Autodesk Inventor part; units mm, degrees
ref_plane "YZ Plane" through (0, 0, 0) normal (1, 0, 0) x (0, 1, 0)
ref_plane "XZ Plane" through (0, 0, 0) normal (0, 1, 0) x (-1, 0, 0)
ref_plane "XY Plane" through (0, 0, 0) normal (0, 0, 1) x (1, 0, 0)
sketch "草圖1" plane through (0, 0, 0) normal (0, 1, 0) x (-1, 0, 0)
  line L0 (-14.2, 4) -> (14.2, 4)
  line L1 (14.2, 4) -> (14.2, -4)
  line L2 (-14.2, -4) -> (-14.2, 4)
  line L3 (-14.2, 4) -> (14.2, -4) construction
  line L4 (14.2, 4) -> (-14.2, -4) construction
  line L5 (-11.2, -4) -> (-11.2, 0)
  line L6 (-11.2, 0) -> (-8.2, 0)
  line L7 (-8.2, 0) -> (-8.2, -4)
  line L8 (0, 7.3969) -> (0, -7.2649)
  line L9 (11.2, -4) -> (11.2, 0)
  line L10 (11.2, 0) -> (8.2, 0)
  line L11 (8.2, 0) -> (8.2, -4)
  line L12 (14.2, -4) -> (11.2, -4)
  line L13 (8.2, -4) -> (-8.2, -4)
  line L14 (-11.2, -4) -> (-14.2, -4)
  point P0 (0, 0)
  dimension "d0" = 4
  dimension "d1" = 8
  dimension "d2" = 16.4
  dimension "d3" = 3
  dimension "d5" = 28.4
extrude "擠出1" add sketch "草圖1" along normal blind 3
equation "\"d5\" = d2 + 4 * d3"
properties part number "upper support"
Could you check a few things on this model? Use its own coordinates, in mm. A direction names the side the tool comes from. Give positions to 0.01 mm unless a question says otherwise; leave off trailing zeros. Write each loop counter-clockwise with the first axis right and the second up, starting at its lowest first coordinate (ties: lowest second). Pieces come first, ordered by that corner, then holes. Notation, with made-up numbers: (17.5, 52.25) -> (39.5, 52.25) arc R20 cw to (39.5, 88.25) -> close; hole circle Ø4 at (72.25, 52). An arc over 180 degrees is marked (long way). Write each question's results on one line, items separated by ' | '. Start each with the question number.
Q1. Suppose I cut it at B-B, the plane y = 2.55. List the corners of the cut face in (x, z) for me, and give its area (3 significant figures).
Q2. Which directions (+Z, -Z, +X, -X, +Y, -Y) give clear straight access to the entire face, cutting with the end or side of a thin tool? Please do faces 4 (the face through (-13, 1, -4)), 5 (the face through (-11.2, 1, -2)).
Q3. We'd pull the mould along X, two halves only. Please class faces 1 (the face through (8.2, 1, -2)), 2 (the face through (0, 3, 0)), 3 (the face through (14.2, 1, 0)): +X half, -X half, draft (parallel to the pull), parting line (faces both ways), or undercut.
Q4. Suppose I cut it at C-C, the plane x = -10. List the corners of the cut face in (y, z) for me, and give its area (3 significant figures).
Q5. Suppose I cut it at A-A, the plane z = -2.25. List the corners of the cut face in (x, y) for me.
Q6. I need wall thicknesses on probe 1 along X at (y, z) = (0.85, -2.5); probe 2 along Z at (x, y) = (9, 2.4). Which ranges of each line are inside material? Lowest first, please.
Outcome:
1) outline: (-14.2, -4) -> (-11.2, -4) -> (-11.2, 0) -> (-8.2, 0) -> (-8.2, -4) -> (8.2, -4) -> (8.2, 0) -> (11.2, 0) -> (11.2, -4) -> (14.2, -4) -> (14.2, 4) -> (-14.2, 4) -> close | area: 203 mm2
2) face 4: -Z, +X, -X, +Y, -Y | face 5: -Z, +Y, -Y
3) face 1: undercut | face 2: draft | face 3: +X half
4) outline: (0, 0) -> (3, 0) -> (3, 4) -> (0, 4) -> close | area: 12.0 mm2
5) outline: (-14.2, 0) -> (-11.2, 0) -> (-11.2, 3) -> (-14.2, 3) -> close; (-8.2, 0) -> (8.2, 0) -> (8.2, 3) -> (-8.2, 3) -> close; (11.2, 0) -> (14.2, 0) -> (14.2, 3) -> (11.2, 3) -> close
6) probe 1: -14.2 to -11.2, -8.2 to 8.2, 11.2 to 14.2 | probe 2: 0 to 4
